Autodesk Fusion 360 part; units mm, degrees
sketch "Sketch1" plane through (0, 0, 0) normal (0, 0, 1) x (1, 0, 0)
  line L0 (0, 0) -> (81.3, 0)
  line L1 (81.3, 0) -> (81.3, 15.4)
  line L2 (81.3, 15.4) -> (0, 15.4)
  line L3 (0, 15.4) -> (0, 0)
  dimension "d8" = 81.3
  dimension "d9" = 15.4
extrude "Extrude1" add sketch "Sketch1" along normal blind 5
sketch "Sketch2" plane through (0, 0, 5) normal (0, 0, 1) x (-1, 0, 0)
  line L0 (0, -15.4) -> (0, 0)
  line L1 (0, 0) -> (-81.3, 0)
  line L2 (-81.3, 0) -> (-81.3, -15.4)
  line L3 (-81.3, -15.4) -> (0, -15.4)
  circle A0 centre (-20.65, -7.7) radius 2.6
  circle A1 centre (-20.65, -7.7) radius 5.1
  line L4 (-40.65, -15.4) -> (-40.65, -7.6842) construction
  line L5 (-40.65, -7.7) -> (-81.3, -7.7) construction
  circle A2 centre (-60.65, -7.7) radius 5.1
  circle A3 centre (-60.65, -7.7) radius 2.6
  dimension "d16" = 5.2
  dimension "d18" = 7.7
  dimension "d19" = 10.2
  dimension "d34" = 20
extrude "Extrude2" cut sketch "Sketch2" against normal blind 5 contours A0 | A3
extrude "Extrude3" cut sketch "Sketch2" against normal blind 3.6 contours A1 | A2
sketch "Sketch3" plane through (0, 0, 5) normal (0, 0, 1) x (1, 0, 0)
  line L0 (40.65, 14.9854) -> (40.65, -0.0146) construction
  line L1 (0, 15.4) -> (0, 0) construction
  line L2 (74.3, 15.4) -> (74.3, 13.4)
  line L3 (74.3, 13.4) -> (79.3, 13.4)
  line L4 (79.3, 13.4) -> (79.3, 2)
  line L5 (79.3, 2) -> (74.3, 2)
  line L6 (74.3, 2) -> (74.3, 0)
  line L7 (74.3, 0) -> (81.3, 0)
  line L8 (81.3, 0) -> (81.3, 15.4)
  line L9 (81.3, 15.4) -> (74.3, 15.4)
  line L10 (0, 0) -> (0, 15.4)
  line L11 (2, 13.4) -> (2, 2)
  line L12 (2, 2) -> (7, 2)
  line L13 (7, 13.4) -> (2, 13.4)
  line L14 (7, 0) -> (0, 0)
  line L15 (7, 15.4) -> (7, 13.4)
  line L16 (0, 15.4) -> (7, 15.4)
  line L17 (7, 2) -> (7, 0)
  line L18 (7, 15.4) -> (74.3, 15.4)
  line L19 (74.3, 15.4) -> (74.3, 13.4)
  line L20 (74.3, 13.4) -> (7, 13.4)
  line L21 (7, 13.4) -> (7, 15.4)
  line L22 (74.3, 2) -> (7, 2)
  line L23 (7, 2) -> (7, 0)
  line L24 (7, 0) -> (74.3, 0)
  line L25 (74.3, 0) -> (74.3, 2)
  point P0 (81.3, 0)
  dimension "d24" = 40.65
  dimension "d25" = 2
  dimension "d26" = 15.4
  dimension "d27" = 2
  dimension "d29" = 5
extrude "Extrude4" add sketch "Sketch3" along normal blind 95.16 contours L2 L3 L4 L5 L6 L7 L8 L9 L19 L25 | L10 L11 L12 L13 L14 L15 L16 L17 L21 L23
extrude "Extrude5" add sketch "Sketch3" along normal blind 5 contours L2 L15 L18 L19 L20 L21 | L6 L17 L22 L23 L24 L25
equation "pw = 74.8 mm"
equation "pd = 8.9 mm"
equation "ph = 158.6 mm"
equation "clearance = 1.25 mm"
equation "wall_thick = 2 mm"
equation "outer_w = 2 * clearance + 2 * wall_thick + pw"
equation "outer_d = 2 * clearance + 2 * wall_thick + pd"
equation "d8 = outer_w"
equation "d9 = outer_d"
equation "d18 = outer_d / 2"
equation "d24 = outer_w / 2"
equation "d25 = wall_thick"
equation "d26 = outer_d"
equation "d27 = wall_thick"
equation "d30 = ph * 0.6"

Autodesk Fusion 360 part; units mm, degrees
sketch "Sketch1" plane through (0, 0, 0) normal (0, 0, 1) x (1, 0, 0)
  circle A0 centre (0, 0) radius 62.5
  line L0 (-16.9429, 20.65) -> (-20.65, 16.9429)
  line L1 (-20.65, -16.9429) -> (-16.9429, -20.65)
  line L2 (-16.9429, -20.65) -> (16.9429, -20.65)
  line L3 (16.9429, 20.65) -> (-16.9429, 20.65)
  line L4 (-20.65, 16.9429) -> (-20.65, -16.9429)
  line L5 (20.65, 16.9429) -> (16.9429, 20.65)
  line L6 (16.9429, -20.65) -> (20.65, -16.9429)
  line L7 (20.65, -16.9429) -> (20.65, 16.9429)
  circle A1 centre (0, 0) radius 11.5
  circle A2 centre (-15.5, 15.5) radius 1.35
  circle A3 centre (0, 0) radius 2
  circle A4 centre (0, 0) radius 20.65 construction
  line L8 (0, 0) -> (0, 20.65) construction
  line L9 (0, 0) -> (20.65, 0) construction
  circle A5 centre (15.5, 15.5) radius 1.35
  circle A6 centre (-15.5, -15.5) radius 1.35
  circle A7 centre (15.5, -15.5) radius 1.35
  circle A8 centre (-20, -40) radius 2.6
  circle A9 centre (20, -40) radius 2.6
  dimension "d1" = 125
  dimension "d2" = 23
  dimension "d3" = 2.7
  dimension "d4" = 15.5
  dimension "d5" = 15.5
  dimension "d8" = 5.2
  dimension "d9" = 40
  dimension "d10" = 20
extrude "Extrude1" add sketch "Sketch1" along normal blind 3 contours A0 | L0 L1 L2 L3 L4 L5 L6 L7
Model file for the job. Use its own axes, mm. A direction names the side the tool comes from. Give positions to 0.01 mm unless a question says otherwise; leave off trailing zeros. Write each loop counter-clockwise with the first axis right and the second up, starting at its lowest first coordinate (ties: lowest second). Pieces come first, ordered by that corner, then holes. Notation, with made-up numbers: (38.25, 37) -> (44.25, 37) arc R17 cw to (44.25, 48) -> close; hole circle Ø4 at (-31, -16). An arc over 180 degrees is marked (long way). Write item = value, one per line.
(1) Slice it at A-A, the plane x = 69.5. Give the cut face in (y, z).
Determined:
outline = (0, 5) -> (2, 5) -> (2, 10) -> (0, 10) -> close; (13.4, 5) -> (15.4, 5) -> (15.4, 10) -> (13.4, 10) -> close
(2) Flat gauge pins, fed straight in: P1, Ø7, axis at x = -20, y = -40, coming from the +Z side; P2, Ø1, axis at y = -3, z = 4, coming from the -X side; P3, Ø0.6, axis at y = 15, z = 62, coming from the -X side. Where does each tip first touch, or does it go through?
Determined:
P1 = 5
P2 = -62.45
P3 = 0
(3) Tool access for faces 1 (the face through (-3, -2, 5)), 2 (the face through (-18.8, -37.693, 2.465)), 3 (the face through (6, 6, 5)), 4 (the face through (80, 8, 100.16)), 5 (the face through (8, 14, 5)): list every direction of +Z, -Z, +X, -X, +Y, -Y with a clear straight run to the whole face (end or side of a thin tool).
Determined:
face_1 = +Z, -X, -Y
face_2 = +Z, -Z
face_3 = +Z
face_4 = +Z, +X, -X, +Y, -Y
face_5 = none
(4) Probe line 1 along Y through (x, z) = (29.5, 7); line 2 along X through (y, z) = (14, 25); line 3 along X through (y, z) = (4, 83). List the from-to ranges inside material, lowest first.
Determined:
line_1 = 0 to 2, 13.4 to 15.4
line_2 = 0 to 7, 74.3 to 81.3
line_3 = 0 to 2, 79.3 to 81.3
(5) Slice it at B-B, the plane z = 17.5. Give the cut face in (x, y).
Determined:
outline = (0, 0) -> (7, 0) -> (7, 2) -> (2, 2) -> (2, 13.4) -> (7, 13.4) -> (7, 15.4) -> (0, 15.4) -> close; (74.3, 0) -> (81.3, 0) -> (81.3, 15.4) -> (74.3, 15.4) -> (74.3, 13.4) -> (79.3, 13.4) -> (79.3, 2) -> (74.3, 2) -> close
(6) Mould opens along Y. For faces 6 (the face through (-1, -27, 5)), 7 (the face through (59, 8, 3)), 8 (the face through (4, 15.4, 45)) say: released by +Y, released by -Y, zero draft, split by the parting line, or undercut.
Determined:
face_6 = zero draft
face_7 = undercut
face_8 = released by +Y
(7) Slice it at C-C, the plane y = -40. Give the cut face in (x, z).
Determined:
outline = (-48.02, 0) -> (-22.6, 0) -> (-22.6, 5) -> (-48.02, 5) -> close; (-17.4, 0) -> (17.4, 0) -> (17.4, 5) -> (-17.4, 5) -> close; (22.6, 0) -> (48.02, 0) -> (48.02, 5) -> (22.6, 5) -> close
(8) Slice it at D-D, the plane x = 50. Give the cut face in (y, z).
Determined:
outline = (-37.5, 0) -> (37.5, 0) -> (37.5, 5) -> (15.4, 5) -> (15.4, 10) -> (13.4, 10) -> (13.4, 5) -> (2, 5) -> (2, 10) -> (0, 10) -> (0, 5) -> (-37.5, 5) -> close
